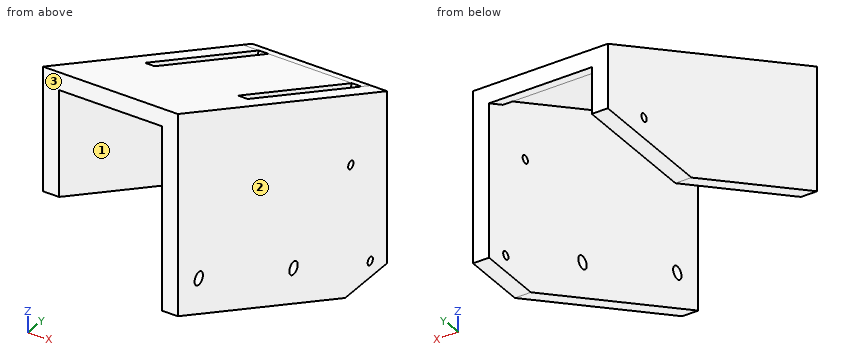
from build123d import *

# Parameters (mm, degrees)
F0_R     = 1.5875
F1_DEPTH = 6.35
F3_DEPTH = 46.99
F4_R     = 1.5875
F5_DEPTH = 6.35
F6_W     = 3.81
F6_H     = 76.2
F7_DEPTH = 6.35
F8_R     = 2.5273
F9_DEPTH = 6.35


with BuildPart() as f1:
    # F0 (on Right) → F1 (new body)
    with BuildSketch(Plane.YZ):
        Polygon((63.5, -63.5), (63.5, 4.2789274143), (-63.5, 63.5), (-63.5, -16.1231419315), (38.1, -63.5), align=None)
        with Locations((53.34, -57.15)):
            Circle(F0_R, mode=Mode.SUBTRACT)
        with Locations((41.5067932579, -12.9878712221)):
            Circle(F0_R, mode=Mode.SUBTRACT)
    extrude(amount=F1_DEPTH)

    # F2 (on face) → F3 (join)
    with BuildSketch(Plane(origin=(0, 0, 0), x_dir=(0, -1, 0), z_dir=(-1, 0, 0))):
        Polygon((11.7045099709, 32.3409165561), (63.5, 56.4935502146), (63.5, 63.5), (9.0208840088, 38.0959710038), align=None)
        Polygon((-63.5, -2.7275223711), (-55.0613195903, 1.2074989287), (-57.7449455523, 6.9625533764), (-63.5, 4.2789274143), align=None)
        Polygon((-55.0613195903, 1.2074989287), (11.7045099709, 32.3409165561), (9.0208840088, 38.0959710038), (-57.7449455523, 6.9625533764), align=None)
    extrude(amount=F3_DEPTH)

    # F4 (on face) → F5 (join)
    with BuildSketch(Plane(origin=(-46.99, 0, 0), x_dir=(0, -1, 0), z_dir=(-1, 0, 0))):
        Polygon((63.5, 63.5), (-63.5, 4.2789274143), (-63.5, -21.1210725857), (-12.7, -21.1210725857), (63.5, 14.4115709657), align=None)
        with Locations((-41.5067932579, -12.9878712221)):
            Circle(F4_R, mode=Mode.SUBTRACT)
    extrude(amount=-F5_DEPTH)

    # F6 (on face) → F7 (cut, through all)
    with BuildSketch(Plane(origin=(0, 12.9804176766, 27.8365955385), x_dir=(1, 0, 0), z_dir=(0, 0.4226182617, 0.906307787))):
        with Locations((-1.905, 11.2921916109)):
            Rectangle(F6_W, F6_H)
        with Locations((-38.735, 11.2921916109)):
            Rectangle(F6_W, F6_H)
    extrude(amount=-F7_DEPTH, mode=Mode.SUBTRACT)

    # F8 (on face) → F9 (cut, through all)
    with BuildSketch(Plane.YZ.offset(6.35)):
        with Locations((-50.8, -8.0323496192)):
            Circle(F8_R)
        with Locations((6.7505444768, -34.8686092397)):
            Circle(F8_R)
    extrude(amount=-F9_DEPTH, mode=Mode.SUBTRACT)


solid = f1.part
The model under review builds one solid part; all positions refer to its coordinate system, in mm. Face numbers are marked on the shaded views. Round coordinates to 2 decimals unless told otherwise and drop trailing zeros. Write each loop counter-clockwise with the first axis right and the second up, starting at its lowest first coordinate (ties: lowest second). Pieces come first, ordered by that corner, then holes. Notation, with made-up numbers: M 14.25,22.5 L 27.25,22.5 A8 ccw 27.25,31.5 Z; hole C -32,38.25 d8. An arc over 180 degrees is marked long. Use a Markdown table: item, result. Add a question column.
Q1. The part is to be moulded in two halves that separate along X. For the marked faces 1, 2 and 3, say which applies: pulls with the +X half, pulls with the -X half, needs draft (parallel to the pull), parting line crosses it, or undercut.
Q2. Insertion check: pin 1 (8 mm diameter, centred on y = -50.8, z = -8.03, fed in from -X); pin 2 (3 mm diameter, centred on x = -8, y = 25, fed in from -Z); pin 3 (1 mm diameter, centred on x = -9, y = 1.5, fed in from +Z); pin 4 (3 mm diameter, centred on y = 6.75, z = -34.87, fed in from -X). Each pin has a flat end and moves straight along its axis. Give the tip position at first contact, or say it passes through.
Q3. We need section A-A, the plane y = 53.34. State the section outline as (x, z) points, plus the area to 3 significant figures.
Q4. We need section C-C, the plane y = 24. State the section outline as (x, z) points, plus the area to 3 significant figures.
Q5. To check wall thickness, follow line 1 (X direction, y = 33, z = 15); line 2 (X direction, y = 30, z = -7); line 3 (X direction, y = -4.5, z = -19). State the ranges of each line that lie inside material, in increasing order.
Q6. We need section D-D, the plane y = -50.8. State the section outline as (x, z) points.
Q7. We need section B-B, the plane x = -28. State the section outline as (y, z) points, plus the area to 3 significant figures.
Findings below:
| question | item | result |
|---|---|---|
| 1 | face 1 | undercut |
| 1 | face 2 | pulls with the +X half |
| 1 | face 3 | needs draft |
| 2 | pin 1 | stops at x = 0 |
| 2 | pin 2 | stops at z = 14.53 |
| 2 | pin 3 | stops at z = 33.42 |
| 2 | pin 4 | passes through |
| 3 | outline | M -46.99,-21.12 L -40.64,-21.12 L -40.64,9.02 L -46.99,9.02 Z; M -36.83,2.01 L -3.81,2.01 L -3.81,9.02 L -36.83,9.02 Z; M 0,-63.5 L 6.35,-63.5 L 6.35,-58.74 L 0,-58.74 Z; M 0,-55.56 L 6.35,-55.56 L 6.35,9.02 L 0,9.02 Z |
| 3 | area | 863 mm² |
| 4 | outline | M -46.99,-21.12 L -40.64,-21.12 L -40.64,22.7 L -46.99,22.7 Z; M -36.83,15.69 L -3.81,15.69 L -3.81,22.7 L -36.83,22.7 Z; M 0,-56.93 L 6.35,-56.93 L 6.35,22.7 L 0,22.7 Z |
| 4 | area | 1,020 mm² |
| 5 | line 1 | x = -46.99 to -40.64, -36.83 to -3.81, 0 to 6.35 |
| 5 | line 2 | x = -46.99 to -40.64, 0 to 6.35 |
| 5 | line 3 | x = 0 to 6.35 |
| 6 | outline | M -46.99,8.49 L -40.64,8.49 L -40.64,50.57 L 0,50.57 L 0,-5.51 L 6.35,-5.51 L 6.35,57.58 L -46.99,57.58 Z; M 0,-22.05 L 6.35,-22.05 L 6.35,-10.56 L 0,-10.56 Z |
| 7 | outline | M -63.5,56.49 L 63.5,-2.73 L 63.5,4.28 L -63.5,63.5 Z |
| 7 | area | 890 mm² |
